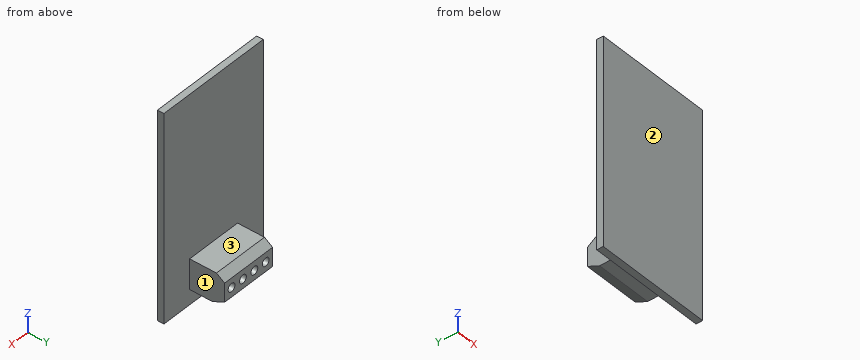
from build123d import *

# Parameters (mm, degrees)
CROQUIS1_W              = 29
CROQUIS1_H              = 50.8
SALIENTE_EXTRUIR1_DEPTH = 1.6
SALIENTE_EXTRUIR2_DEPTH = 7
CROQUIS3_R              = 1
CORTAR_EXTRUIR1_DEPTH   = 3


with BuildPart() as part:
    # Croquis1 → Saliente-Extruir1 (new body)
    with BuildSketch(Plane(origin=(0, 0, 0), x_dir=(1, 0, 0), z_dir=(0, 1, 0))):
        Rectangle(CROQUIS1_W, CROQUIS1_H)
    extrude(amount=SALIENTE_EXTRUIR1_DEPTH)

    # Croquis2 → Saliente-Extruir2 (add, symmetric)
    with BuildSketch(Plane(origin=(0, 0, 0), x_dir=(0, 0, -1), z_dir=(1, 0, 0))):
        Polygon((14.3, 1.6), (14.3, 8.2), (15.7, 10.2), (20.3, 10.2), (21.7, 7.2), (21.7, 1.6), align=None)
    extrude(amount=SALIENTE_EXTRUIR2_DEPTH, both=True)

    # Croquis3 → Cortar-Extruir1 (cut)
    with BuildSketch(Plane(origin=(0, 10.2, 0), x_dir=(1, 0, 0), z_dir=(0, 1, 0))):
        with Locations((-5, 18)):
            Circle(CROQUIS3_R)
        with Locations((-1.67, 18)):
            Circle(CROQUIS3_R)
        with Locations((1.66, 18)):
            Circle(CROQUIS3_R)
        with Locations((4.99, 18)):
            Circle(CROQUIS3_R)
    extrude(amount=-CORTAR_EXTRUIR1_DEPTH, mode=Mode.SUBTRACT)


solid = part.part
Can you work these out from the model? Positions are in its coordinate system, mm. Face numbers are marked on the shaded views. A direction names the side the tool comes from. Round coordinates to 2 decimals unless told otherwise and drop trailing zeros. Write each loop counter-clockwise with the first axis right and the second up, starting at its lowest first coordinate (ties: lowest second). Pieces come first, ordered by that corner, then holes. Notation, with made-up numbers: (78, -31) - (105, -31) arc R17 ccw to (105, -23) - close; hole circle Ø1 at (-40, -34). An arc over 180 degrees is marked (long way). Write each question's results on one line, items separated by ' | '. Start each with the question number.
1) Please list where these lines run through material, in increasing order: line 1 (X direction, y = 8.75, z = -18); line 2 (Y direction, x = -6.25, z = -6); line 3 (Z direction, x = -5.25, y = 2).
2) Which directions (+Z, -Z, +X, -X, +Y, -Y) give clear straight access to the entire face, cutting with the end or side of a thin tool? Please do the marked faces 1, 2 and 3.
3) Suppose I cut it at A-A (x = 3.25). List the corners of the cut face in (y, z) for me.
4) Suppose I cut it at C-C (x = -5). List the corners of the cut face in (y, z) for me.
5) For pin 1 Ø1 at (x, z) = (-1.5, -18) entering from +Y; pin 2 Ø2 at (y, z) = (5.5, -18.5) entering from +X; pin 3 Ø3.5 at (x, y) = (-3, 6.5) entering from +Z, each with a flat end and sliding along its axis, tell me the tip position at first contact or that it passes through.
6) Suppose I cut it at B-B (z = -21). List the corners of the cut face in (x, y) for me.
7) Suppose I cut it at D-D (y = 6.25). List the corners of the cut face in (x, z) for me.
Here are the results:
1) line 1: x = -7 to -6, -4 to -2.67, -0.67 to 0.66, 2.66 to 3.99, 5.99 to 7 | line 2: y = 0 to 1.6 | line 3: z = -21.7 to -14.3
2) face 1: +Z, -Z, +X, +Y | face 2: +Z, -Z, +X, -X, -Y | face 3: +Z, +X, -X, +Y
3) outline: (0, -25.4) - (1.6, -25.4) - (1.6, -21.7) - (7.2, -21.7) - (10.2, -20.3) - (10.2, -15.7) - (8.2, -14.3) - (1.6, -14.3) - (1.6, 25.4) - (0, 25.4) - close
4) outline: (0, -25.4) - (1.6, -25.4) - (1.6, -21.7) - (7.2, -21.7) - (10.2, -20.3) - (10.2, -19) - (7.2, -19) - (7.2, -17) - (10.2, -17) - (10.2, -15.7) - (8.2, -14.3) - (1.6, -14.3) - (1.6, 25.4) - (0, 25.4) - close
5) pin 1: stops at y = 7.2 | pin 2: stops at x = 7 | pin 3: stops at z = -14.3
6) outline: (-14.5, 0) - (14.5, 0) - (14.5, 1.6) - (7, 1.6) - (7, 8.7) - (-7, 8.7) - (-7, 1.6) - (-14.5, 1.6) - close
7) outline: (-7, -21.7) - (7, -21.7) - (7, -14.3) - (-7, -14.3) - close
